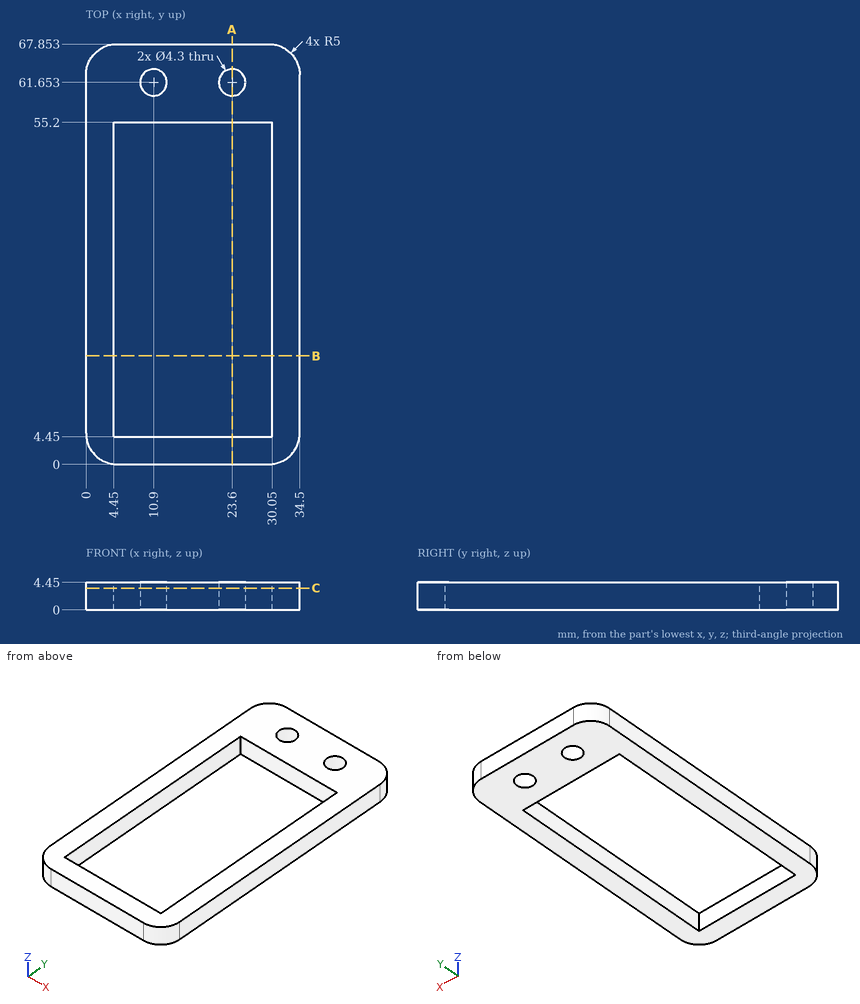
Design review of the part shown in the three views and the two pictorial views. Dimensions are in mm from the part's minimum x, y and z. Round coordinates to 2 decimals unless told otherwise and drop trailing zeros. Write each loop counter-clockwise with the first axis right and the second up, starting at its lowest first coordinate (ties: lowest second). Pieces come first, ordered by that corner, then holes.
Item 1: We need section A-A on x = 23.6. Write out the cut boundary in (y, z), and give its area (3 significant figures).
Item 2: Clearance check with flat-ended pins moving along their axes: pin 1 Ø10 at (x, y) = (30, 33.5) entering from -Z; pin 2 Ø1.5 at (x, z) = (4, 1) entering from +Y. State where each tip first meets the part, or that it passes through.
Item 3: We need section B-B on y = 17.5. Write out the cut boundary in (x, z).
Item 4: We need section C-C on z = 3.5. Write out the cut boundary in (x, y).
Item 5: For probe 1 along Y at (x, z) = (23.6, 1.55); probe 2 along Y at (x, z) = (8.5, 4.1); probe 3 along X at (y, z) = (52.5, 0.55), list the stretches that pass through material, from the lowest coordinate up.
Returned:
1. outline: (0, 0) - (4.45, 0) - (4.45, 4.45) - (0, 4.45) - close; (55.2, 0) - (59.5, 0) - (59.5, 4.45) - (55.2, 4.45) - close; (63.8, 0) - (67.85, 0) - (67.85, 4.45) - (63.8, 4.45) - close
1. area: 57.0 mm2
2. pin 1: stops at z = 0
2. pin 2: stops at y = 67.85
3. outline: (0, 0) - (4.45, 0) - (4.45, 4.45) - (0, 4.45) - close; (30.05, 0) - (34.5, 0) - (34.5, 4.45) - (30.05, 4.45) - close
4. outline: (0, 5) arc R5 ccw to (5, 0) - (29.5, 0) arc R5 ccw to (34.5, 5) - (34.5, 62.85) arc R5 ccw to (29.5, 67.85) - (5, 67.85) arc R5 ccw to (0, 62.85) - close; hole (4.45, 4.45) - (30.05, 4.45) - (30.05, 55.2) - (4.45, 55.2) - close; hole circle Ø4.3 at (10.9, 61.65); hole circle Ø4.3 at (23.6, 61.65)
5. probe 1: y = 0 to 4.45, 55.2 to 59.5, 63.8 to 67.85
5. probe 2: y = 0 to 4.45, 55.2 to 67.85
5. probe 3: x = 0 to 4.45, 30.05 to 34.5
